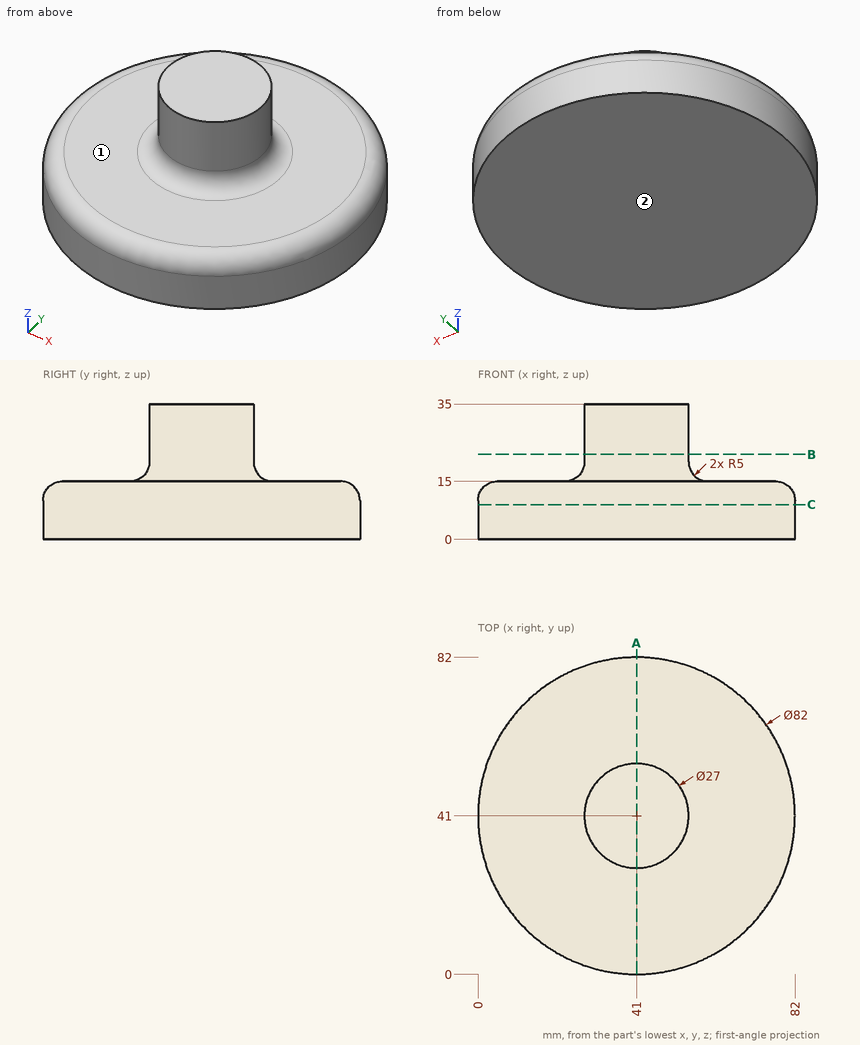
For this review, use the dimensioned drawing (mm, ordinates from the lowest corner) and the shaded views. A direction names the side the tool comes from. Give positions to 0.01 mm unless a question says otherwise; leave off trailing zeros. Order: outer loops, then holes, each group sorted by start corner. A loop starts at its lowest first (then second) coordinate and runs counter-clockwise, first axis right, second up.
1) Wall thickness on line 1 (Z direction, x = 56.5, y = 72.5); line 2 (Z direction, x = 58.5, y = 41.5); line 3 (X direction, y = 76, z = 2): over which ranges is each line inside the solid? List them lowest first.
2) Take a section at B-B (z = 22). Give the boundary of the cut face in (x, y).
3) Insertion check: pin 1 (1.5 mm diameter, centred on y = 13.5, z = 9.5, fed in from +X); pin 2 (8 mm diameter, centred on x = 56.5, y = 16, fed in from +Z); pin 3 (2 mm diameter, centred on x = 48.5, z = 12.5, fed in from +Y); pin 4 (5 mm diameter, centred on x = 55.5, y = 39, fed in from +Z). Each pin has a flat end and moves straight along its axis. Give the tip position at first contact, or say it passes through.
4) Take a section at C-C (z = 9). Give the boundary of the cut face in (x, y).
5) For the marked faces 1 and 2, list the 3-axis set-ups (+Z, -Z, +X, -X, +Y, -Y) from which the entire face can be reached by the end or side of a thin tool; tool diameter is ignored.
6) Take a section at A-A (x = 41). Give the boundary of the cut face in (y, z).
Derived:
1. line 1: z = 0 to 15
1. line 2: z = 0 to 15.1
1. line 3: x = 19.65 to 62.35
2. outline: circle Ø27 at (41, 41)
3. pin 1: stops at x = 72.07
3. pin 2: stops at z = 15
3. pin 3: stops at y = 81.12
3. pin 4: stops at z = 35
4. outline: circle Ø82 at (41, 41)
5. face 1: +Z
5. face 2: -Z, +X, -X, +Y, -Y
6. outline: (0, 0) - (82, 0) - (82, 10) arc R5 ccw to (77, 15) - (59.5, 15) arc R5 cw to (54.5, 20) - (54.5, 35) - (27.5, 35) - (27.5, 20) arc R5 cw to (22.5, 15) - (5, 15) arc R5 ccw to (0, 10) - close
